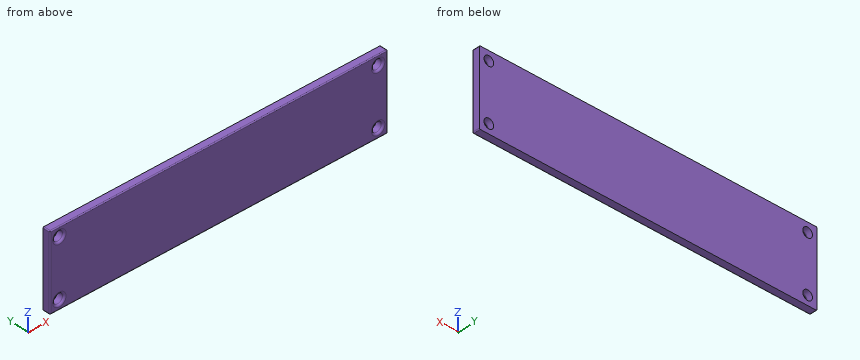
from build123d import *

# Parameters (mm, degrees)
F0_W     = 180
F0_H     = 40
F0_R     = 2.5751263091
F1_DEPTH = 4
F2_R     = 1
F3_R     = 0.5


# Not quite as in the source:
# - a feature names something its author has since deleted; it is built from what else it names


with BuildPart() as f1:
    # F0 (on Front) → F1 (new body)
    with BuildSketch(Plane.XZ):
        Rectangle(F0_W, F0_H)
        with Locations((-85, -15)):
            Circle(F0_R, mode=Mode.SUBTRACT)
        with Locations((85, -15)):
            Circle(F0_R, mode=Mode.SUBTRACT)
        with Locations((-85, 15)):
            Circle(F0_R, mode=Mode.SUBTRACT)
        with Locations((85, 15)):
            Circle(F0_R, mode=Mode.SUBTRACT)
    extrude(amount=F1_DEPTH)

    # F2
    f2_edges = [f1.edges().sort_by_distance(p)[0] for p in [
        (-87.575126, -4, 15),
        (-87.575126, -4, -15),
        (82.424874, -4, 15),
        (82.424874, -4, -15),
    ]]
    fillet(f2_edges, radius=F2_R)

    # F3
    f3_edges = [f1.edges().sort_by_distance(p)[0] for p in [
        (0, -4, 20),
        (-90, -4, 0),
        (0, -4, -20),
        (90, -4, 0),
        (-90, -2, 20),
        (-90, -2, -20),
        (90, -2, 20),
        (90, -2, -20),
    ]]
    fillet(f3_edges, radius=F3_R)


solid = f1.part
Geometry: final body of the model. Coordinates: model frame, mm. Give positions to 0.01 mm unless a question says otherwise; leave off trailing zeros. Write each loop counter-clockwise with the first axis right and the second up, starting at its lowest first coordinate (ties: lowest second). Pieces come first, ordered by that corner, then holes.
(1) Ray query, line 1 (Z direction, x = -85, y = -1.1); line 2 (X direction, y = -3.55, z = -14); line 3 (X direction, y = -3, z = 15.5). Return the intervals inside material, ascending.
(2) Cut plane A-A, the plane x = 85. Return loops of the section in (y, z).
(3) First-contact query: P1, Ø6, axis at x = -85, z = -15, coming from the -Y side; P2, Ø6.5, axis at x = 85, z = -15, coming from the -Y side. Flat tips, straight axial feed; report the tip coordinate or a pass-through.
(4) Cut plane B-B, the plane z = -15. Return loops of the section in (x, y), then the cut area to 3 significant figures.
Values follow:
1. line 1: z = -20 to -17.58, -12.42 to 12.42, 17.58 to 20
1. line 2: x = -90 to -87.55, -82.45 to 82.45, 87.55 to 90
1. line 3: x = -90 to -87.53, -82.47 to 82.47, 87.53 to 90
2. outline: (-4, -19.5) arc R0.5 ccw to (-3.5, -20) - (0, -20) - (0, -17.58) - (-3, -17.58) arc R1 ccw to (-4, -18.58) - close; (-4, -11.42) arc R1 ccw to (-3, -12.42) - (0, -12.42) - (0, 12.42) - (-3, 12.42) arc R1 ccw to (-4, 11.42) - close; (-4, 18.58) arc R1 ccw to (-3, 17.58) - (0, 17.58) - (0, 20) - (-3.5, 20) arc R0.5 ccw to (-4, 19.5) - close
3. P1: stops at y = -3.82
3. P2: stops at y = -3.95
4. outline: (-90, -3.5) arc R0.5 ccw to (-89.5, -4) - (-88.58, -4) arc R1 ccw to (-87.58, -3) - (-87.58, 0) - (-90, 0) - close; (-82.42, -3) arc R1 ccw to (-81.42, -4) - (81.42, -4) arc R1 ccw to (82.42, -3) - (82.42, 0) - (-82.42, 0) - close; (87.58, -3) arc R1 ccw to (88.58, -4) - (89.5, -4) arc R0.5 ccw to (90, -3.5) - (90, 0) - (87.58, 0) - close
4. area: 678 mm2
